Autodesk Inventor part; units mm, degrees
ref_plane "YZ Plane" through (0, 0, 0) normal (1, 0, 0) x (0, 1, 0)
ref_plane "XZ Plane" through (0, 0, 0) normal (0, 1, 0) x (-1, 0, 0)
ref_plane "XY Plane" through (0, 0, 0) normal (0, 0, 1) x (1, 0, 0)
sketch "Szkic1" plane through (0, 0, 0) normal (0, 0, 1) x (1, 0, 0)
  arc A0 (85.75, 216.779101) -> (95.75, 226.779101) centre (85.75, 226.779101) ccw
  line L0 (85.75, 216.779101) -> (83.25, 216.779101)
  arc A1 (83.25, 216.779101) -> (53.25, 186.779101) centre (83.25, 186.779101) ccw
  line L1 (53.25, 186.779101) -> (53.25, -39)
  arc A2 (46.25, -46) -> (53.25, -39) centre (46.25, -39) ccw
  line L2 (-1.25, -46) -> (46.25, -46)
  arc A3 (-8.916667, 45.356612) -> (-1.25, -46) centre (-1.25, 0) ccw
  arc A4 (-8.916667, 45.356612) -> (-7.25, 47.328638) centre (-9.25, 47.328638) ccw
  line L3 (-7.25, 400) -> (-7.25, 47.328638)
  arc A5 (27.038691, 446) -> (-7.25, 400) centre (40.75, 400) ccw
  line L4 (85.75, 446) -> (27.038691, 446)
  arc A6 (95.75, 436) -> (85.75, 446) centre (85.75, 436) ccw
  line L5 (95.75, 226.779101) -> (95.75, 436)
  circle A7 centre (46.75, 361.06) radius 2
  circle A8 centre (40.75, 400) radius 23.333333
  circle A9 centre (85.75, 438.7) radius 2
  circle A10 centre (85.75, 361.06) radius 2
  circle A11 centre (46.75, 438.7) radius 2
  circle A12 centre (-10.958284, -29.879026) radius 2.1
  circle A13 centre (-32.666667, 0) radius 2.1
  circle A14 centre (24.166617, -18.466253) radius 2.1
  circle A15 centre (-10.958284, 29.879026) radius 2.1
  circle A16 centre (24.166617, 18.466253) radius 2.1
  circle A17 centre (-1.25, 0) radius 23.333333
  circle A18 centre (1.75, 302.77336) radius 2.25
  circle A19 centre (1.75, 237.161813) radius 2.25
  circle A20 centre (43.75, 127.673594) radius 2
  circle A21 centre (4.75, -38.7) radius 2
  circle A22 centre (4.75, 38.94) radius 2
  circle A23 centre (4.75, 127.673594) radius 2
  circle A24 centre (43.75, -38.7) radius 2
  circle A25 centre (43.75, 38.94) radius 2
  circle A26 centre (45.25, 237.161813) radius 2
  circle A27 centre (88.75, 302.77336) radius 2
  circle A28 centre (45.25, 302.77336) radius 2
  circle A29 centre (88.75, 237.161813) radius 2
  circle A30 centre (66.166617, 381.533747) radius 2.1
  circle A31 centre (66.166617, 418.466253) radius 2.1
  circle A32 centre (31.041716, 370.120974) radius 2.1
  circle A33 centre (31.041716, 429.879026) radius 2.1
  circle A34 centre (9.333333, 400) radius 2.1
  circle A35 centre (88.75, 237.161813) radius 6
  circle A36 centre (1.75, 237.161813) radius 6
  line L6 (88.75, 231.161813) -> (1.75, 231.161813)
  line L7 (88.75, 243.161813) -> (1.75, 243.161813)
  point P0 (0, 0)
  dimension "d0" = 12
  dimension "d1" = 12
extrude "Wyciągnięcie proste1" add sketch "Szkic1" along normal blind 22 contours A35 | A35 L6 A36 L7 | A36
sketch "Szkic2" plane through (1.75, 231.161813, 0) normal (0, -1, 0) x (1, 0, 0)
  circle A0 centre (64.5, 22.5) radius 16
  circle A1 centre (64.5, 22.5) radius 15.927206
  circle A2 centre (22.5, 22.5) radius 16
  circle A3 centre (64.5, 22.5) radius 16
  point P0 (-1.75, 0)
sketch "Szkic2 outline for Wyciągnięcie proste2" plane through (1.75, 231.161813, 0) normal (0, -1, 0) x (1, 0, 0)
  circle A0 centre (22.5, 22.5) radius 16
  circle A1 centre (64.5, 22.5) radius 15.927206
extrude "Wyciągnięcie proste2" cut sketch "Szkic2 outline for Wyciągnięcie proste2" against normal through all
properties part number "uchwyt_na_silniki_v2"
Could you check a few things on this model? Use its own coordinates, in mm. Give positions to 0.01 mm unless a question says otherwise; leave off trailing zeros. Order: outer loops, then holes, each group sorted by start corner. A loop starts at its lowest first (then second) coordinate and runs counter-clockwise, first axis right, second up.
1. Suppose I cut it at D-D (y = 232.5). List the corners of the cut face in (x, z) for me, plus the area to 3 significant figures.
2. I need wall thicknesses on L1, parallel to X at y = 234.5, z = 18; L2, parallel to X at y = 236.25, z = 14.75; L3, parallel to Y at x = 1.75, z = 10.5. Which ranges of each line are inside material? Lowest first, please.
3. Will this pin go through, and if not, where does the flat tip stop? P1, Ø12, axis at x = 77.5, z = 15.5, coming from the -Y side.
4. Suppose I cut it at A-A (x = 45.25). List the corners of the cut face in (y, z) for me, plus the area to 3 significant figures.
5. Suppose I cut it at C-C (z = 15). List the corners of the cut face in (x, y) for me.
6. Suppose I cut it at B-B (z = 11.25). List the corners of the cut face in (x, y) for me, plus the area to 3 significant figures.
7. We'd pull the mould along Y, two halves only. Please class faces 1 (the cylindrical face through (-0.036, 238.531, 10.846)), 2 (the flat face through (46, 243.162, 8)), 3 (the flat face through (87, 239, 22)), 4 (the cylindrical face through (46.173, 238.936, 10.846)): pulls with the +Y half, pulls with the -Y half, needs draft (parallel to the pull), parting line crosses it, or undercut.
Solved:
1. outline: (-2.03, 0) - (92.53, 0) - (92.53, 22) - (82.17, 22) arc R15.93 cw to (50.33, 22) - (40.24, 22) arc R16 cw to (8.26, 22) - (-2.03, 22) - close
1. area: 1,310 mm2
2. L1: x = -3.63 to 8.9, 39.6 to 50.97, 81.53 to 94.13
2. L2: x = -4.18 to -0.31, 3.81 to 10.25, 38.25 to 43.47, 47.03 to 52.34, 80.16 to 86.97, 90.53 to 94.68
2. L3: y = 231.16 to 234.91, 239.41 to 243.16
3. P1: stops at y = 231.16
4. outline: (231.16, 0) - (235.16, 0) - (235.16, 22) - (231.16, 22) - close; (239.16, 0) - (243.16, 0) - (243.16, 22) - (239.16, 22) - close
4. area: 176 mm2
5. outline: (1.75, 231.16) - (10.12, 231.16) - (10.12, 243.16) - (1.75, 243.16) arc R6 ccw to start; (38.38, 231.16) - (52.2, 231.16) - (52.2, 243.16) - (38.38, 243.16) - close; (80.3, 231.16) - (88.75, 231.16) arc R6 ccw to (88.75, 243.16) - (80.3, 243.16) - close; hole circle Ø4.5 at (1.75, 237.16); hole circle Ø4 at (45.25, 237.16); hole circle Ø4 at (88.75, 237.16)
6. outline: (1.75, 231.16) - (12.87, 231.16) - (12.87, 243.16) - (1.75, 243.16) arc R6 ccw to start; (35.63, 231.16) - (54.98, 231.16) - (54.98, 243.16) - (35.63, 243.16) - close; (77.52, 231.16) - (88.75, 231.16) arc R6 ccw to (88.75, 243.16) - (77.52, 243.16) - close; hole circle Ø4.5 at (1.75, 237.16); hole circle Ø4 at (45.25, 237.16); hole circle Ø4 at (88.75, 237.16)
6. area: 572 mm2
7. face 1: undercut
7. face 2: pulls with the +Y half
7. face 3: needs draft
7. face 4: undercut
